from build123d import *

# Parameters (mm, degrees)
ESBO_O1_R                = 3.175
RESSALTO_EXTRUS_O1_DEPTH = 22.4
CHANFRO1_SIZE            = 0.5
ESBO_O3_W                = 2.89827535
ESBO_O3_H                = 0.35
CORTE_EXTRUS_O1_DEPTH    = 16
ESBO_O4_R                = 0.75
CORTE_EXTRUS_O2_DEPTH    = 3


with BuildPart() as part:
    # Esboço1 → Ressalto-extrusão1 (new body)
    with BuildSketch(Plane(origin=(0, 0, 0), x_dir=(0, 0, -1), z_dir=(1, 0, 0))):
        Circle(ESBO_O1_R)
    extrude(amount=RESSALTO_EXTRUS_O1_DEPTH)

    # Chanfro1
    chanfro1_edges = [part.edges().sort_by_distance(p)[0] for p in [
        (22.4, 0, 3.175),
    ]]
    chamfer(chanfro1_edges, length=CHANFRO1_SIZE)

    # Esboço3 → Corte-extrusão1 (cut)
    with BuildSketch(Plane(origin=(22.4, 0, 0), x_dir=(0, 0, -1), z_dir=(1, 0, 0))):
        with Locations((0, 3)):
            Rectangle(ESBO_O3_W, ESBO_O3_H)
    extrude(amount=-CORTE_EXTRUS_O1_DEPTH, mode=Mode.SUBTRACT)

    # Esboço4 → Corte-extrusão2 (cut)
    with BuildSketch(Plane(origin=(22.4, 0, 0), x_dir=(0, 0, -1), z_dir=(1, 0, 0))):
        Circle(ESBO_O4_R)
    extrude(amount=-CORTE_EXTRUS_O2_DEPTH, mode=Mode.SUBTRACT)


solid = part.part
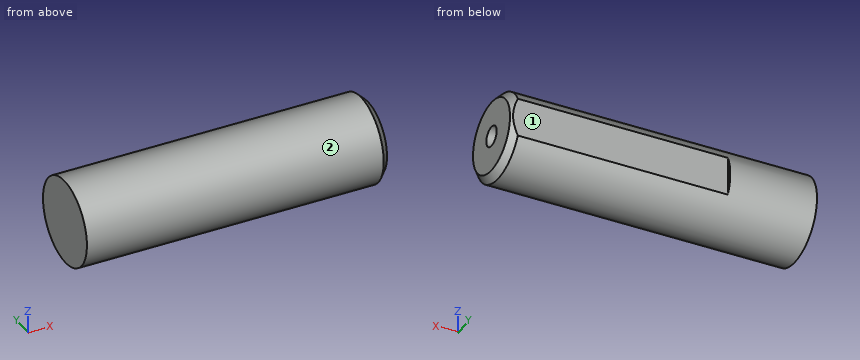
Work out the finished part from the listing and answer in its coordinate system (mm). Face numbers are marked on the shaded views. A direction names the side the tool comes from. Give positions to 0.01 mm unless a question says otherwise; leave off trailing zeros. Loops run counter-clockwise (first coordinate to the right, second up) from the corner with the lowest first, then second, coordinate; pieces in that order, holes last. Notation, with made-up numbers: (71, 13.25) -> (92, 13.25) arc R35 cw to (92, 51.25) -> close; hole circle Ø7 at (81.25, 8.25). An arc over 180 degrees is marked (long way). Use a Markdown table: item, result. Add a question column.
1) Consider line 1 along Y through (x, z) = (20.1, 0) (3 decimals); line 2 along Y through (x, z) = (18, 0) (3 decimals); line 3 along X through (y, z) = (-0.5, 0.25). Determine where each line is inside the solid, lowest interval first.
2) Each of these flat-tipped pins is pushed along its axis until it touches: P1, Ø1.5, axis at x = 17, z = -1, coming from the -Y side; P2, Ø1.5, axis at x = 17.5, z = -1, coming from the +Y side (3 decimals). Where does it stop, or does it pass through?
3) The part is cut by section C-C, the plane x = 18.25. Determine the outline of the cut face in (y, z) (3 decimals), plus the area to 3 significant figures.
4) Which of the six approach directions +Z, -Z, +X, -X, +Y, -Y give full straight-line access (tool end or side, diameter ignored) to the marked faces 1 and 2?
5) The part is cut by section B-B, the plane z = 0. Determine the outline of the cut face in (x, y) (3 decimals), plus the area to 3 significant figures.
6) The part is cut by section A-A, the plane y = 0. Determine the outline of the cut face in (x, z) (3 decimals).
Reported:
| question | item | result |
|---|---|---|
| 1 | line 1 | y = -3.175 to -0.75, 0.75 to 2.825 |
| 1 | line 2 | y = -3.175 to 2.825 |
| 1 | line 3 | x = 0 to 19.4 |
| 2 | P1 | stops at y = -3.17 |
| 2 | P2 | stops at y = 2.825 |
| 3 | outline | (2.825, -1.449) -> (2.825, 1.449) arc R3.175 ccw (long way) to start |
| 3 | area | 31.0 mm^2 |
| 4 | face 1 | +Z, -Z, +X, +Y |
| 4 | face 2 | +X, -X |
| 5 | outline | (0, -3.175) -> (21.9, -3.175) -> (22.4, -2.675) -> (22.4, -0.75) -> (19.4, -0.75) -> (19.4, 0.75) -> (22.4, 0.75) -> (22.4, 2.675) -> (22.25, 2.825) -> (6.4, 2.825) -> (6.4, 3.175) -> (0, 3.175) -> close |
| 5 | area | 132 mm^2 |
| 6 | outline | (0, -3.175) -> (21.9, -3.175) -> (22.4, -2.675) -> (22.4, -0.75) -> (19.4, -0.75) -> (19.4, 0.75) -> (22.4, 0.75) -> (22.4, 2.675) -> (21.9, 3.175) -> (0, 3.175) -> close |
